from build123d import *


with BuildPart() as part:
    # Sketch1 → Revolve1 (revolve)
    with BuildSketch(Plane(origin=(0, 0, 0), x_dir=(0, 0, -1), z_dir=(1, 0, 0)), mode=Mode.PRIVATE) as revolve1_sk:
        with BuildLine():
            Line((0.291524109, 49.911154557), (2.625, 49.2))
            Line((2.625, 49.2), (2.625, 46.5))
            Line((2.625, 46.5), (1.4, 46.5))
            ThreePointArc((1.4, 46.5), (0, 46.846700168), (-1.4, 46.5))
            Line((-1.4, 46.5), (-2.625, 46.5))
            Line((-2.625, 46.5), (-2.625, 49.2))
            Line((-2.625, 49.2), (-0.291524109, 49.911154557))
            ThreePointArc((-0.291524109, 49.911154557), (0, 49.954591076), (0.291524109, 49.911154557))
        make_face()
    revolve(revolve1_sk.sketch.rotate(Axis((0, 0, 0), (0, 0, -1)), 90), axis=Axis((0, 0, 0), (0, 0, -1)))


solid = part.part
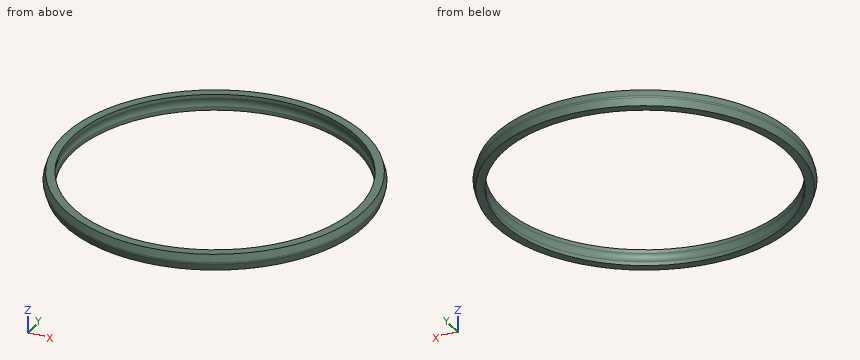
Geometry: final body of the model. Coordinates: model frame, mm. Coordinates: 2 decimals unless noted, no trailing zeros. Loops run counter-clockwise (first coordinate to the right, second up) from the corner with the lowest first, then second, coordinate; pieces in that order, holes last. Notation, with made-up numbers: M -12,19 L 2,19 A22 ccw 2,27 Z; hole C -22,70 d10. An arc over 180 degrees is marked long. One line per item, written item: value. Start each with the question number.
1) Material intervals for L1, parallel to X at y = 10.5, z = -2.2; L2, parallel to X at y = -42, z = 1.75; L3, parallel to Y at x = 0, z = -1.7, sorted ascending. Write a range as from..to.
2) Pin query (flat end, axial travel): P1, Ø1, axis at x = 36.5, z = -1, coming from the -Y side; P2, Ø1.5, axis at y = 3, z = -1, coming from the -X side. Return the tip coordinate at first contact, or that it passes through.
3) Cut plane A-A (y = 0). Return loops of the section in (x, z) (3 decimals).
Evaluation:
1. L1: -48.2..-45.3, 45.3..48.2
1. L2: -26.13..-19.96, 19.96..26.13
1. L3: -49.48..-46.5, 46.5..49.48
2. P1: y = -34.3
2. P2: x = -49.84
3. outline: M -49.911,-0.292 L -49.2,-2.625 L -46.5,-2.625 L -46.5,-1.4 A3 cw -46.5,1.4 L -46.5,2.625 L -49.2,2.625 L -49.911,0.292 A1 ccw Z; M 46.5,-2.625 L 49.2,-2.625 L 49.911,-0.292 A1 ccw 49.911,0.292 L 49.2,2.625 L 46.5,2.625 L 46.5,1.4 A3 cw 46.5,-1.4 Z
